from build123d import *

# Parameters (mm, degrees)
SKETCH1_R           = 2.2
BOSS_EXTRUDE1_DEPTH = 3
BOSS_EXTRUDE2_DEPTH = 3


with BuildPart() as part:
    # Sketch1 → Boss-Extrude1 (new body)
    with BuildSketch(Plane(origin=(0, 0, 0), x_dir=(1, 0, 0), z_dir=(0, 1, 0))):
        with Locations(Location((0, 0, 0), (0, 0, 270))):
            Circle(SKETCH1_R)
    boss_extrude1 = extrude(amount=BOSS_EXTRUDE1_DEPTH)

    # Sketch2 → Boss-Extrude2 (add)
    with BuildSketch(Plane(origin=(0, 3, 0), x_dir=(1, 0, 0), z_dir=(0, 1, 0))):
        Polygon((-1.558845727, 2.7), (-3.117691454, 0), (-1.558845727, -2.7), (1.558845727, -2.7), (3.117691454, 0), (1.558845727, 2.7), align=None)
    boss_extrude2 = extrude(amount=BOSS_EXTRUDE2_DEPTH)

    # Mirror1: Boss-Extrude1, Boss-Extrude2 across plane
    add(boss_extrude1.mirror(Plane.ZX))
    add(boss_extrude2.mirror(Plane.ZX))


solid = part.part
Input: part model. Units: mm. Frame: model coordinates. Coordinates: 2 decimals unless noted, no trailing zeros. Order: outer loops, then holes, each group sorted by start corner. A loop starts at its lowest first (then second) coordinate and runs counter-clockwise, first axis right, second up.
1. Cut plane B-B, the plane y = 0.75. Return loops of the section in (x, z), plus the area to 3 significant figures.
Checked values:
outline: circle Ø4.4 at (0, 0)
area: 15.2 mm2
2. Draft query along Y for faces 1 (the cylindrical face through (2.18, 0.04, -0.29)), 2 (the flat face through (0, -6, 0)), 3 (the flat face through (0, -4, -2.7)). Return one class per face: +Y half, -Y half, draft (parallel to the pull), parting line (faces both ways), or undercut.
Checked values:
face 1: undercut
face 2: -Y half
face 3: draft
3. Cut plane D-D, the plane y = 4.75. Return loops of the section in (x, z).
Checked values:
outline: (-3.12, 0) - (-1.56, -2.7) - (1.56, -2.7) - (3.12, 0) - (1.56, 2.7) - (-1.56, 2.7) - close
4. Ray query, line 1 along Y through (x, z) = (-2.5, -0.1); line 2 along X through (y, z) = (2, 1.55); line 3 along X through (y, z) = (-2.75, 0). Return the intervals inside material, ascending.
Checked values:
line 1: y = -6 to -3, 3 to 6
line 2: x = -1.56 to 1.56
line 3: x = -2.2 to 2.2
5. Cut plane C-C, the plane z = 1.8. Return loops of the section in (x, y).
Checked values:
outline: (-2.08, -6) - (2.08, -6) - (2.08, -3) - (1.26, -3) - (1.26, 3) - (2.08, 3) - (2.08, 6) - (-2.08, 6) - (-2.08, 3) - (-1.26, 3) - (-1.26, -3) - (-2.08, -3) - close
6. Cut plane A-A, the plane x = 0. Return loops of the section in (y, z).
Checked values:
outline: (-6, -2.7) - (-3, -2.7) - (-3, -2.2) - (3, -2.2) - (3, -2.7) - (6, -2.7) - (6, 2.7) - (3, 2.7) - (3, 2.2) - (-3, 2.2) - (-3, 2.7) - (-6, 2.7) - close
7. Contact query for a flat-ended pin moving along its axis: P1, Ø1, axis at y = -0.5, z = -2, coming from the +X side. Output: stop coordinate, or through.
Checked values:
P1: stops at x = 1.61
